Autodesk Inventor part; units mm, degrees
ref_plane "YZ Plane" through (0, 0, 0) normal (1, 0, 0) x (0, 1, 0)
ref_plane "XZ Plane" through (0, 0, 0) normal (0, 1, 0) x (-1, 0, 0)
ref_plane "XY Plane" through (0, 0, 0) normal (0, 0, 1) x (1, 0, 0)
sketch "スケッチ1" plane through (0, 0, 0) normal (0, 1, 0) x (-1, 0, 0)
  circle A0 centre (0, 0) radius 125
  dimension "d0" = 250
extrude "押し出し1" add sketch "スケッチ1" along normal blind 4
sketch "スケッチ2" plane through (0, 4, 0) normal (0, 1, 0) x (1, 0, 0)
  line L0 (75, -84.411) -> (-75, -84.411)
  line L1 (-75, -84.411) -> (-75, 95.589)
  line L2 (-75, 95.589) -> (75, 95.589)
  line L3 (75, 95.589) -> (75, -84.411)
  line L4 (75, -84.411) -> (-75, 95.589) construction
  line L5 (-75, -84.411) -> (75, 95.589) construction
  circle A0 centre (0, 0) radius 121.5
  line L6 (0, 0) -> (0, -125) construction
  circle A1 centre (0, 0) radius 125
  line L7 (0, 0) -> (108.2532, 62.5) construction
  line L8 (0, 0) -> (-108.2532, 62.5) construction
  circle A2 centre (-16.75, 82.589) radius 4.1
  point P0 (0, 5.589)
  dimension "d3" = 150
  dimension "d4" = 180
  dimension "d5" = 243
  dimension "d8" = 360
  dimension "d12" = 16.75
  dimension "d13" = 13
  dimension "d14" = 8.2
extrude "押し出し2" cut sketch "スケッチ2" against normal blind 4 contours A2
sketch "スケッチ4" plane through (0, 4, 0) normal (0, 1, 0) x (1, 0, 0)
  circle A0 centre (0, 0) radius 121.5
  line L0 (75, -84.411) -> (-75, -84.411)
  line L1 (-75, -84.411) -> (-75, 95.589)
  line L2 (-75, 95.589) -> (75, 95.589)
  line L3 (75, 95.589) -> (75, -84.411)
  line L4 (75, -84.411) -> (-75, 95.589) construction
  line L5 (-75, -84.411) -> (75, 95.589) construction
  line L6 (0, 0) -> (0, -29.9183)
  point P0 (0, 5.589)
  point P1 (69, -54.411)
  point P2 (69, 5.589)
  point P3 (69, 65.589)
  point P4 (-69, -54.411)
  point P5 (-69, 5.589)
  point P6 (-69, 65.589)
  dimension "d17" = 243
  dimension "d18" = 150
  dimension "d19" = 180
  dimension "d20" = 30
  dimension "d21" = 6
  dimension "d22" = 60
  dimension "d23" = 60
hole "穴1" at (69, 4, 54.411) at (69, 4, -5.589) at (69, 4, -65.589) at (-69, 4, -65.589) at (-69, 4, -5.589) at (-69, 4, 54.411) direction (0, -1, 0) diameter 3.2 end through all
properties part number "中間台1" material "MDF 中密度繊維ボード"
Work out the finished part from the listing and answer in its coordinate system (mm). Give positions to 0.01 mm unless a question says otherwise; leave off trailing zeros. Write each loop counter-clockwise with the first axis right and the second up, starting at its lowest first coordinate (ties: lowest second). Pieces come first, ordered by that corner, then holes.
Q1. The part is cut by section B-B on x = -16.75. Give the vertices of the cut face in (y, z).
Answer:
outline: (0, -123.87) - (4, -123.87) - (4, -86.69) - (0, -86.69) - close; (0, -78.49) - (4, -78.49) - (4, 123.87) - (0, 123.87) - close
Q2. Straight lines are drawn through the part: L1, parallel to Z at x = 69, y = 0.9; L2, parallel to X at y = 1.05, z = -67; L3, parallel to Z at x = -16.75, y = 1.2. For each, find the intervals that lie inside material, in ascending order.
Answer:
L1: z = -104.23 to -67.19, -63.99 to -7.19, -3.99 to 52.81, 56.01 to 104.23
L2: x = -105.53 to -69.75, -68.25 to 68.25, 69.75 to 105.53
L3: z = -123.87 to -86.69, -78.49 to 123.87
Q3. The part is cut by section A-A on y = 2.45. Give the vertices of the cut face in (x, z), and give its area (3 significant figures).
Answer:
outline: circle Ø250 at (0, 0); hole circle Ø3.2 at (-69, -65.59); hole circle Ø3.2 at (-69, -5.59); hole circle Ø3.2 at (-69, 54.41); hole circle Ø8.2 at (-16.75, -82.59); hole circle Ø3.2 at (69, -65.59); hole circle Ø3.2 at (69, -5.59); hole circle Ø3.2 at (69, 54.41)
area: 49,000 mm2
Q4. The part is cut by section D-D on z = -58. Give the vertices of the cut face in (x, y).
Answer:
outline: (-110.73, 0) - (110.73, 0) - (110.73, 4) - (-110.73, 4) - close
Q5. The part is cut by section C-C on x = 59. Give the vertices of the cut face in (y, z).
Answer:
outline: (0, -110.2) - (4, -110.2) - (4, 110.2) - (0, 110.2) - close
Q6. For a pull along X with two mould halves and no side action, classify faces 1 (the face through (2, 0, 2)), 2 (the face through (-17.284, 2.028, -86.654)), 3 (the face through (124.88, 1.97, -5.5)) as released by +X, released by -X, zero draft, split by the parting line, or undercut.
Answer:
face 1: zero draft
face 2: undercut
face 3: split by the parting line
Q7. Given pin 1 (2 mm diameter, centred on y = 1.5, z = 86, fed in from -X); pin 2 (12 mm diameter, centred on x = 10, z = 31, fed in from -Y); pin 3 (1.5 mm diameter, centred on x = -96, y = 1, fed in from +Z), each flat-ended and moving along its own axis, determine where each tip first touches the part or whether it passes through.
Answer:
pin 1: stops at x = -91.65
pin 2: stops at y = 0
pin 3: stops at z = 80.95
